Input: part model. Units: mm. Frame: model coordinates. A direction names the side the tool comes from. Coordinates: 2 decimals unless noted, no trailing zeros. Write each loop counter-clockwise with the first axis right and the second up, starting at its lowest first coordinate (ties: lowest second). Pieces come first, ordered by that corner, then holes. Notation, with made-up numbers: M -11,83.5 L 43,83.5 A14 cw 43,109.5 Z; hole C 4.5,63 d11. An arc over 180 degrees is marked long. Write each question's results on one line, items separated by ' | '. Start each with the question number.
1. Set-up query: faces 1 (the cylindrical face through (11.923, 3.755, 15.226)), 2 (the cylindrical face through (11.894, 1.154, 4.091)), 3 (the flat face through (3.875, 12, 58)). Return all of +Z, -Z, +X, -X, +Y, -Y with unobstructed straight access to the full face (end or side cutting, diameter ignored); none if empty.
2. First-contact query: pin 1 (2 mm diameter, centred on x = 3.5, y = -4, fed in from -Z); pin 2 (6 mm diameter, centred on x = -0.5, z = 52, fed in from +Y) (3 decimals); pin 3 (1 mm diameter, centred on y = 12, z = 67, fed in from -X); pin 4 (5 mm diameter, centred on y = -1, z = 22.5, fed in from -X). Flat tips, straight axial feed; report the tip coordinate or a pass-through.
3. Ray query, probe 1 along Z at (x, y) = (12, 3); probe 2 along X at (y, z) = (0.75, 42.5); probe 3 along Z at (x, y) = (-6.25, -11.5). Return the intervals inside material, ascending.
4. Section query D-D, the plane z = 30.5. Output: boundary loops of the cut face in (x, y) (3 decimals).
5. Pull-direction query (X, two-part tool) for faces 4 (the flat face through (0, 12, 26)), 5 (the cylindrical face through (11.923, 3.755, 99.476)), 6 (the flat face through (0, 0, 0)); classes: +X half, -X half, draft (parallel to the pull), parting line (faces both ways), or undercut.
6. Section query C-C, the plane z = 101.5. Output: boundary loops of the cut face in (x, y).
```python
from build123d import *

# Parameters (mm, degrees)
SKETCH1_R                      = 12.5
BOSS_EXTRUDE1_DEPTH            = 115
BOSS_EXTRUDE2_DEPTH            = 31.5
BOSS_EXTRUDE2_DEPTH_BACK       = 31.5
SKETCH2_R                      = 14.5
CUT_EXTRUDE1_REACH             = 63.047
SKETCH3_W                      = 7.75
SKETCH3_H                      = 7.75
CUT_EXTRUDE1_DIRECTION_2_REACH = 63.047
SKETCH4_W                      = 1.1
SKETCH4_H                      = 1.3
CHAMFER1_SIZE                  = 1


with BuildPart() as part:
    # Sketch1 → Boss-Extrude1 (new body)
    with BuildSketch(Plane.XY):
        Circle(SKETCH1_R)
    extrude(amount=BOSS_EXTRUDE1_DEPTH)

    # Sketch2 → Boss-Extrude2 (add, two sides: drawn at the far end of the back side and taken through both)
    with BuildSketch(Plane(origin=(0, 0, 57.5), x_dir=(-1, 0, 0), z_dir=(0, 0, -1)).offset(-BOSS_EXTRUDE2_DEPTH_BACK)):
        Circle(SKETCH2_R)
    extrude(amount=BOSS_EXTRUDE2_DEPTH + BOSS_EXTRUDE2_DEPTH_BACK)

    # Cut-Extrude1: up to this face of the body (flat: up to its plane)
    cut_extrude1_end = Plane(part.part.faces().sort_by_distance((14.089878067, 0, 89))[0])
    # Sketch3 → Cut-Extrude1 (cut, up to the picked face)
    with BuildSketch(Plane(origin=(0, 0, 57.5), x_dir=(-1, 0, 0), z_dir=(0, 0, -1)), mode=Mode.PRIVATE) as cut_extrude1_sk1:
        with Locations((0, 14.5)):
            Rectangle(SKETCH3_W, SKETCH3_H)
    cut_extrude1_tool1 = split(extrude(cut_extrude1_sk1.sketch, amount=-CUT_EXTRUDE1_REACH, mode=Mode.PRIVATE), bisect_by=cut_extrude1_end, keep=Keep.BOTH, mode=Mode.PRIVATE)
    add(cut_extrude1_tool1.solids().sort_by(Axis((0, 14.5, 57.5), (0, 0, 1)))[0], mode=Mode.SUBTRACT)

    # Cut-Extrude1 direction 2: up to this face of the body (flat: up to its plane)
    cut_extrude1_direction_2_end = Plane(part.part.faces().sort_by_distance((14.089878067, 0, 26))[0])
    # Sketch3 → Cut-Extrude1 direction 2 (cut, up to the picked face)
    with BuildSketch(Plane(origin=(0, 0, 57.5), x_dir=(-1, 0, 0), z_dir=(0, 0, -1)), mode=Mode.PRIVATE) as cut_extrude1_direction_2_sk1:
        with Locations((0, 14.5)):
            Rectangle(SKETCH3_W, SKETCH3_H)
    cut_extrude1_direction_2_tool1 = split(extrude(cut_extrude1_direction_2_sk1.sketch, amount=CUT_EXTRUDE1_DIRECTION_2_REACH, mode=Mode.PRIVATE), bisect_by=cut_extrude1_direction_2_end, keep=Keep.BOTH, mode=Mode.PRIVATE)
    add(cut_extrude1_direction_2_tool1.solids().sort_by(Axis((0, 14.5, 57.5), (0, 0, -1)))[0], mode=Mode.SUBTRACT)

    # Sketch4 → Cut-Revolve1 (revolve, cut)
    with BuildSketch(Plane(origin=(0, 0, 0), x_dir=(1, 0, 0), z_dir=(0, 1, 0)), mode=Mode.PRIVATE) as cut_revolve1_sk:
        with Locations((-12.5, -4.1)):
            Rectangle(SKETCH4_W, SKETCH4_H)
    cut_revolve1 = revolve(cut_revolve1_sk.sketch.rotate(Axis((0, 0, 0), (0, 0, 1)), 288.059230491), axis=Axis((0, 0, 0), (0, 0, 1)), mode=Mode.SUBTRACT)

    # Mirror1: Cut-Revolve1 across plane
    add(cut_revolve1.mirror(Plane(origin=(0, 0, 57.5), x_dir=(1, 0, 0), z_dir=(0, 0, -1))), mode=Mode.SUBTRACT)

    # Chamfer1
    chamfer1_edges = [part.edges().sort_by_distance(p)[0] for p in [
        (-12.5, 0, 0),
        (-12.5, 0, 115),
    ]]
    chamfer(chamfer1_edges, length=CHAMFER1_SIZE)


solid = part.part
```
Answer:
1) face 1: -Z | face 2: none | face 3: +Y
2) pin 1: z = 0 | pin 2: y = 10.625 | pin 3: x = -8.83 | pin 4: x = -12.5
3) probe 1: 0.87 to 3.45, 4.75 to 110.25, 111.55 to 114.13 | probe 2: -14.48 to 14.48 | probe 3: 26 to 89
4) outline: M -3.875,10.625 L -3.875,13.973 A14.5 ccw long 3.875,13.973 L 3.875,10.625 Z
5) face 4: undercut | face 5: parting line | face 6: draft
6) outline: C 0,0 d25
